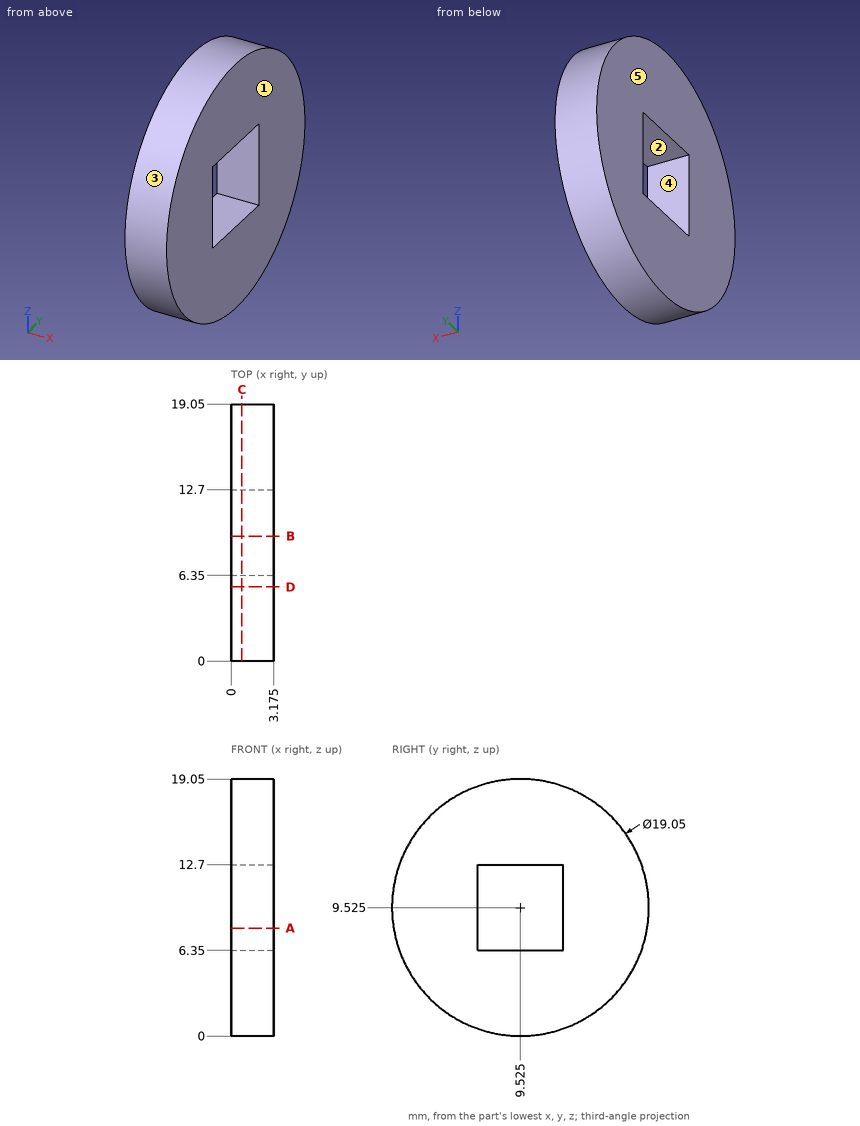
Input: dimensioned drawing with shaded views. Units: mm. Origin: part minimum x, y, z. A direction names the side the tool comes from. Round coordinates to 2 decimals unless told otherwise and drop trailing zeros. Loops run counter-clockwise (first coordinate to the right, second up) from the corner with the lowest first, then second, coordinate; pieces in that order, holes last. Notation, with made-up numbers: (27.5, 38) -> (80.5, 38) arc R4 ccw to (80.5, 42) -> close; hole circle Ø10 at (61.5, -35.5). An arc over 180 degrees is marked (long way). Answer as a JSON object with one key per item and string values. Group by question number.
Q1. Ray query, line 1 (Z direction, x = 0.65, y = 6.75); line 2 (Y direction, x = 2.45, z = 8.5); line 3 (Z direction, x = 0.8, y = 6.5). Return the intervals inside material, ascending. Write a range as from..to.
Q2. Section query A-A (z = 8). Output: boundary loops of the cut face in (x, y) (3 decimals), plus the area to 3 significant figures.
Q3. Contact query for a flat-ended pin moving along its axis: P1, Ø1, axis at x = 1, y = 12, coming from the -Z side. Output: stop coordinate, or through.
Q4. Section query C-C (x = 0.8). Output: boundary loops of the cut face in (y, z) (3 decimals).
Q5. Section query D-D (y = 5.5). Output: boundary loops of the cut face in (x, z) (3 decimals).
Q6. Access query for the marked faces 4 and 5. Directions: +Z, -Z, +X, -X, +Y, -Y. A direction counts if a zero-diameter tool reaches every point of the face in a straight line with its end or side. Return the directions, or none.
Q7. Mould query, pull axis Z, two halves, no side actions, for the marked faces 1, 2 and 3. Classes: pulls with the +Z half, pulls with the -Z half, needs draft (parallel to the pull), parting line crosses it, or undercut.
Q8. Section query B-B (y = 9.25). Output: boundary loops of the cut face in (x, z) (3 decimals), plus the area to 3 significant figures.
Completed:
{
 "1": {"line 1": "0.41..6.35, 12.7..18.64", "line 2": "0.06..6.35, 12.7..18.99", "line 3": "0.49..6.35, 12.7..18.56"},
 "2": {"outline": "(0, 0.123) -> (3.175, 0.123) -> (3.175, 6.35) -> (0, 6.35) -> close; (0, 12.7) -> (3.175, 12.7) -> (3.175, 18.927) -> (0, 18.927) -> close", "area": "39.5 mm²"},
 "3": {"P1": "z = 0.21"},
 "4": {"outline": "circle Ø19.05 at (9.525, 9.525); hole (6.35, 6.35) -> (12.7, 6.35) -> (12.7, 12.7) -> (6.35, 12.7) -> close"},
 "5": {"outline": "(0, 0.892) -> (3.175, 0.892) -> (3.175, 18.158) -> (0, 18.158) -> close"},
 "6": {"face 4": "+X, -X", "face 5": "+Z, -Z, -X, +Y, -Y"},
 "7": {"face 1": "needs draft", "face 2": "undercut", "face 3": "parting line crosses it"},
 "8": {"outline": "(0, 0.004) -> (3.175, 0.004) -> (3.175, 6.35) -> (0, 6.35) -> close; (0, 12.7) -> (3.175, 12.7) -> (3.175, 19.046) -> (0, 19.046) -> close", "area": "40.3 mm²"}
}
